Build history of the part. All positions in model axes, mm. Face numbers are marked on the shaded views. A direction names the side the tool comes from. Give positions to 0.01 mm unless a question says otherwise; leave off trailing zeros. One line per question, with ' | ' between items. Start each with the question number.
(1) Pin check, flat tips, straight feed: P1, Ø1, axis at x = -2, y = 4.5, coming from the -Z side; P2, Ø8, axis at x = -17, y = -15, coming from the +Z side; P3, Ø1, axis at y = 4.5, z = 5, coming from the -X side. Stop position of each tip, or through.
(2) Tool access for the marked faces 1 and 2: list every direction of +Z, -Z, +X, -X, +Y, -Y with a clear straight run to the whole face (end or side of a thin tool).
(3) Drill centre lines: probe 1 along Z at (x, y) = (-15.5, -3.5); probe 2 along X at (y, z) = (-5.5, 24); probe 3 along X at (y, z) = (10, -8.5). Where is each one in solid material? Low to high. Write a range as from..to.
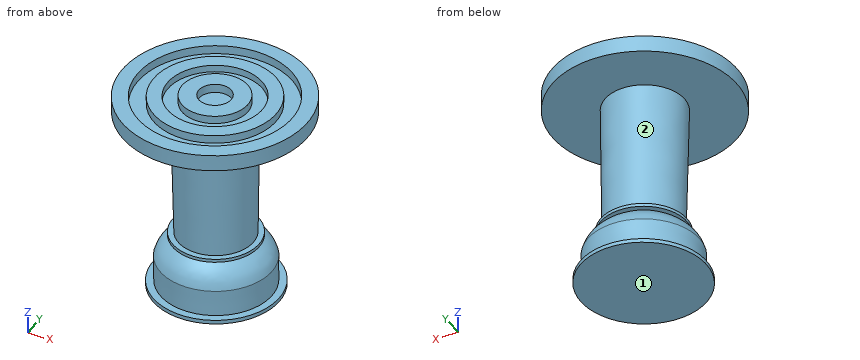
from build123d import *


with BuildPart() as f1:
    # F0 (on Front) → F1 (revolve)
    with BuildSketch(Plane.XZ):
        with BuildLine():
            Line((4.5143341753, -4.3006491445), (4.8665297218, 29.8076476902))
            Line((4.8665297218, 29.8076476902), (15.1177551597, 29.8076476902))
            Line((15.1177551597, 29.8076476902), (18.4809826314, 29.8076476902))
            Line((18.4809826314, 29.8076476902), (18.4809826314, 34.0604297817))
            Line((18.4809826314, 34.0604297817), (14.5479189232, 34.0604297817))
            Line((14.5479189232, 34.0604297817), (14.5479189232, 31.8417809904))
            Line((14.5479189232, 31.8417809904), (10.413158685, 31.8417809904))
            Line((10.413158685, 31.8417809904), (10.413158685, 33.9595861733))
            Line((10.413158685, 33.9595861733), (6.7826374434, 33.9595861733))
            Line((6.7826374434, 33.9595861733), (6.7826374434, 32.1443229914))
            Line((6.7826374434, 32.1443229914), (3.0619536992, 32.1443229914))
            Line((3.0619536992, 32.1443229914), (3.0619536992, 34.2173911631))
            Line((3.0619536992, 34.2173911631), (-1.2554875575, 34.2173911631))
            Line((-1.2554875575, 34.2173911631), (-1.2554875575, 31.9387428463))
            Line((-1.2554875575, 31.9387428463), (-5.4606664926, 31.9387428463))
            Line((-5.4606664926, 31.9387428463), (-5.117402412, -18.8897587359))
            Line((-5.117402412, -18.8897587359), (11.2336110324, -18.8897587359))
            Line((11.2336110324, -18.8897587359), (11.2336110324, -17.870362848))
            Line((11.2336110324, -17.870362848), (9.3235522509, -17.870362848))
            Line((9.3235522509, -17.870362848), (9.3235522509, -10.993424803))
            add(Edge.make_bspline(
                [(4.4993474148, -5.128914956), (4.9297158996, -5.4351701742), (5.788696219, -6.0464305579), (7.0241461042, -7.0064449477), (8.0186108337, -8.1847141484), (8.7726157993, -9.3142207885), (9.131741148, -10.4088020701), (9.3235522509, -10.993424803)],
                knots=[0, 0, 0, 0, 0.2018948913, 0.402965701, 0.6005252736, 0.7866380413, 1, 1, 1, 1], degree=3))
            Line((4.4993474148, -5.128914956), (5.9968610294, -5.128914956))
            Line((5.9968610294, -5.128914956), (5.9968610294, -4.3006491445))
            Line((5.9968610294, -4.3006491445), (4.5143341753, -4.3006491445))
        make_face()
    revolve(axis=Axis((-5.2890344523, 0, 6.5244920552), (0.0067532239, 0, -0.9999771967)))


solid = f1.part
Results:
1) P1: stops at z = -18.91 | P2: stops at z = 33.87 | P3: stops at x = -14.33
2) face 1: -Z, +X | face 2: none
3) probe 1: z = -19.03..-6.12, -5.27..-4.44, 29.67..32 | probe 2: x = -14.02..3.2 | probe 3: x = -13.95..3.7
